```python
from build123d import *

# Parameters (mm, degrees)
SKETCH1_R           = 1.5
SKETCH1_R_2         = 1.25
BOSS_EXTRUDE1_DEPTH = 3.175


with BuildPart() as part:
    # Sketch1 → Boss-Extrude1 (new body)
    with BuildSketch(Plane(origin=(0, 0, 0), x_dir=(1, 0, 0), z_dir=(0, 1, 0))):
        with BuildLine():
            Line((-44.45, 75), (10, 75))
            Line((10, 75), (10, -15))
            ThreePointArc((10, -15), (-35.153948529, -15.397564184), (-79.768950839, -8.430592532))
            Line((-79.768950839, -8.430592532), (-44.45, 75))
        make_face()
        Circle(SKETCH1_R, mode=Mode.SUBTRACT)
        with Locations((-30, 0)):
            Circle(SKETCH1_R, mode=Mode.SUBTRACT)
        with Locations((-30, 30)):
            Circle(SKETCH1_R, mode=Mode.SUBTRACT)
        with Locations((-30, 60)):
            Circle(SKETCH1_R, mode=Mode.SUBTRACT)
        with Locations((0, 60)):
            Circle(SKETCH1_R, mode=Mode.SUBTRACT)
        with Locations((0, 30)):
            Circle(SKETCH1_R, mode=Mode.SUBTRACT)
        with Locations((-46.7, 63.8)):
            Circle(SKETCH1_R_2, mode=Mode.SUBTRACT)
        with Locations((1.5, 69.95)):
            Circle(SKETCH1_R_2, mode=Mode.SUBTRACT)
        with Locations((-31.5, 39.7)):
            Circle(SKETCH1_R_2, mode=Mode.SUBTRACT)
        with Locations((-3.6, 39.7)):
            Circle(SKETCH1_R_2, mode=Mode.SUBTRACT)
        with Locations((-46.7, -11.1)):
            Circle(SKETCH1_R_2, mode=Mode.SUBTRACT)
        with Locations((1.5, -12.4)):
            Circle(SKETCH1_R_2, mode=Mode.SUBTRACT)
    extrude(amount=BOSS_EXTRUDE1_DEPTH)


solid = part.part
```
Can you work these out from the model? Positions are in its coordinate system, mm. Coordinates: 2 decimals unless noted, no trailing zeros. Loops run counter-clockwise (first coordinate to the right, second up) from the corner with the lowest first, then second, coordinate; pieces in that order, holes last.
1) For pin 1 (2.5 mm diameter, centred on x = 0, z = -60, fed in from -Y), with a flat end and sliding along its axis, tell me the tip position at first contact or that it passes through.
2) Imagine slicing it at B-B on x = -46.7. List the corners of the cut face in (y, z) for me (3 decimals), plus the area to 3 significant figures.
3) Imagine slicing it at A-A on z = 0. List the corners of the cut face in (x, y) for me (3 decimals).
4) I need wall thicknesses on probe 1 along Z at (x, y) = (-29, 1.3); probe 2 along Z at (x, y) = (-30, 2.25); probe 3 along X at (y, z) = (2.45, -30). Which ranges of each line are inside material? Lowest first, please.
5) Imagine slicing it at C-C on y = 1.2. State how many separate pieces and enclosed holes the cut face has, plus the area to 3 significant figures.
6) Thinking about a two-plate mould opening in Z: for faces 1 (the cylindrical face through (-30.923, 1.565, -38.591)), 2 (the flat face through (-62.357, 1.565, -32.701)), 3 (the flat face through (10, 2, -31)), 4 (the cylindrical face through (-0.195, 1.565, -31.487)), which applies, pulls with the +Z half, pulls with the -Z half, needs draft (parallel to the pull), parting line crosses it, or undercut?
7) Imagine slicing it at D-D on x = -3.6. List the corners of the cut face in (y, z) for me (3 decimals), plus the area to 3 significant figures.
Completed:
1. pin 1: passes through
2. outline: (0, -69.685) - (3.175, -69.685) - (3.175, -65.05) - (0, -65.05) - close; (0, -62.55) - (3.175, -62.55) - (3.175, 9.85) - (0, 9.85) - close; (0, 12.35) - (3.175, 12.35) - (3.175, 14.308) - (0, 14.308) - close
2. area: 251 mm2
3. outline: (-76.2, 0) - (-31.5, 0) - (-31.5, 3.175) - (-76.2, 3.175) - close; (-28.5, 0) - (-1.5, 0) - (-1.5, 3.175) - (-28.5, 3.175) - close; (1.5, 0) - (10, 0) - (10, 3.175) - (1.5, 3.175) - close
4. probe 1: z = -75 to -61.12, -58.88 to -31.12, -28.88 to -1.12, 1.12 to 15.78
4. probe 2: z = -75 to -61.5, -58.5 to -31.5, -28.5 to -1.5, 1.5 to 15.73
4. probe 3: x = -63.5 to -31.5, -28.5 to -1.5, 1.5 to 10
5. separate pieces: 1
5. enclosed holes: 12
5. area: 6,460 mm2
6. face 1: undercut
6. face 2: pulls with the -Z half
6. face 3: needs draft
6. face 4: undercut
7. outline: (0, -75) - (3.175, -75) - (3.175, -40.95) - (0, -40.95) - close; (0, -38.45) - (3.175, -38.45) - (3.175, 15.899) - (0, 15.899) - close
7. area: 281 mm2
